from build123d import *

# Parameters (mm, degrees)
ESQUISSE1_R             = 6.25
BOSS_EXTRU_1_DEPTH      = 24
ENL_V_MAT_EXTRU_1_DEPTH = 12
ESQUISSE5_W             = 2
ESQUISSE5_H             = 2
ENL_V_MAT_EXTRU_3_DEPTH = 10


with BuildPart() as part:
    # Esquisse1 → Boss.-Extru.1 (new body)
    with BuildSketch(Plane(origin=(0, 0, 0), x_dir=(1, 0, 0), z_dir=(0, 1, 0))):
        with Locations(Location((0, 0, 0), (0, 0, 270))):
            Circle(ESQUISSE1_R)
    extrude(amount=BOSS_EXTRU_1_DEPTH)

    # Esquisse4 → Enlèv. mat.-Extru.1 (cut)
    with BuildSketch(Plane.XZ):
        with BuildLine():
            Line((1.671638418, 3.075), (1.671638418, -3.075))
            ThreePointArc((1.671638418, -3.075), (-3.5, 0), (1.671638418, 3.075))
        make_face()
    extrude(amount=-ENL_V_MAT_EXTRU_1_DEPTH, mode=Mode.SUBTRACT)

    # Esquisse5 → Enlèv. mat.-Extru.3 (cut)
    with BuildSketch(Plane(origin=(0, 24, 0), x_dir=(1, 0, 0), z_dir=(0, 1, 0))):
        with BuildLine():
            Line((-1, 1), (1, 1))
            Line((1, 1), (1, 2.291287847))
            ThreePointArc((1, 2.291287847), (0, 2.5), (-1, 2.291287847))
            Line((-1, 2.291287847), (-1, 1))
        make_face()
        with BuildLine():
            Line((1, 1), (1, -1))
            Line((1, -1), (2.291287847, -1))
            ThreePointArc((2.291287847, -1), (2.5, 0), (2.291287847, 1))
            Line((2.291287847, 1), (1, 1))
        make_face()
        with BuildLine():
            Line((-2.291287847, -1), (-1, -1))
            Line((-1, -1), (-1, 1))
            Line((-1, 1), (-2.291287847, 1))
            ThreePointArc((-2.291287847, 1), (-2.5, 0), (-2.291287847, -1))
        make_face()
        with BuildLine():
            ThreePointArc((-1, -2.291287847), (0, -2.5), (1, -2.291287847))
            Line((1, -2.291287847), (1, -1))
            Line((1, -1), (-1, -1))
            Line((-1, -1), (-1, -2.291287847))
        make_face()
        Rectangle(ESQUISSE5_W, ESQUISSE5_H)
    extrude(amount=-ENL_V_MAT_EXTRU_3_DEPTH, mode=Mode.SUBTRACT)


solid = part.part
Could you check a few things on this model? Use its own coordinates, in mm. A direction names the side the tool comes from. Round coordinates to 2 decimals unless told otherwise and drop trailing zeros. Write each loop counter-clockwise with the first axis right and the second up, starting at its lowest first coordinate (ties: lowest second). Pieces come first, ordered by that corner, then holes. Notation, with made-up numbers: (8.25, 53.25) - (14.25, 53.25) arc R15 ccw to (14.25, 76.25) - close; hole circle Ø9 at (69, 57). An arc over 180 degrees is marked (long way). Use a Markdown table: item, result.
Q1. I want a section at D-D (y = 2.5). List the corners of the cut face in (x, z) for me (3 decimals), plus the area to 3 significant figures.
Output values:
| item | result |
|---|---|
| outline | circle Ø12.5 at (0, 0); hole (1.672, -3.075) - (1.672, 3.075) arc R3.5 ccw (long way) to start |
| area | 92.2 mm2 |
Q2. Please list where these lines run through material, in increasing order: L1, parallel to X at y = 7, z = 0; L2, parallel to X at y = 22.75, z = -2; L3, parallel to Z at x = 1.5, y = 11.
Output values:
| item | result |
|---|---|
| L1 | -6.25 to -3.5, 1.67 to 6.25 |
| L2 | -5.92 to -1, 1 to 5.92 |
| L3 | -6.07 to -3.16, 3.16 to 6.07 |
Q3. Thinking about a two-plate mould opening in X: for faces 1 (the cylindrical face through (1.88, 11.83, 5.96)), 2 (the flat face through (-1.3, 24, 1.3)), 3 (the flat face through (0, 14, 0)), which applies, released by +X, released by -X, zero draft, split by the parting line, or undercut?
Output values:
| item | result |
|---|---|
| face 1 | split by the parting line |
| face 2 | zero draft |
| face 3 | undercut |
Q4. For faces 4 (the flat face through (1.672, 6, 0)), 5 (the flat face through (3, 0, 0)), 6 (the cylindrical face through (-2.5, 19.1, 0)), which set-ups out of +Z, -Z, +X, -X, +Y, -Y let a thin tool reach every point of the face, with its end or its side?
Output values:
| item | result |
|---|---|
| face 4 | -Y |
| face 5 | +Z, -Z, +X, -X, -Y |
| face 6 | +Y |
Q5. I want a section at B-B (z = 0). List the corners of the cut face in (x, y) for me.
Output values:
| item | result |
|---|---|
| outline | (-6.25, 0) - (-3.5, 0) - (-3.5, 12) - (1.67, 12) - (1.67, 0) - (6.25, 0) - (6.25, 24) - (2.5, 24) - (2.5, 14) - (-2.5, 14) - (-2.5, 24) - (-6.25, 24) - close |
Q6. I want a section at C-C (x = 0.75). List the corners of the cut face in (y, z) for me.
Output values:
| item | result |
|---|---|
| outline | (0, -6.2) - (24, -6.2) - (24, -2.38) - (14, -2.38) - (14, 2.38) - (24, 2.38) - (24, 6.2) - (0, 6.2) - (0, 3.42) - (12, 3.42) - (12, -3.42) - (0, -3.42) - close |
Q7. I want a section at A-A (y = 19.25). List the corners of the cut face in (x, z) for me.
Output values:
| item | result |
|---|---|
| outline | circle Ø12.5 at (0, 0); hole (-2.29, -1) - (-1, -1) - (-1, -2.29) arc R2.5 ccw to (1, -2.29) - (1, -1) - (2.29, -1) arc R2.5 ccw to (2.29, 1) - (1, 1) - (1, 2.29) arc R2.5 ccw to (-1, 2.29) - (-1, 1) - (-2.29, 1) arc R2.5 ccw to start |
Q8. For pin 1 (0.6 mm diameter, centred on y = 19, z = -2, fed in from -X); pin 2 (0.6 mm diameter, centred on x = -1.5, y = 18, fed in from +Z); pin 3 (3 mm diameter, centred on y = 14.5, z = -4, fed in from +X), each with a flat end and sliding along its axis, tell me the tip position at first contact or that it passes through.
Output values:
| item | result |
|---|---|
| pin 1 | x = -6.01 |
| pin 2 | z = 6.13 |
| pin 3 | x = 5.73 |
